Geometry check sheet. Reference: the model listing, model coordinates, mm. Face numbers are marked on the shaded views. A direction names the side the tool comes from. Coordinates: 2 decimals unless noted, no trailing zeros. Write each loop counter-clockwise with the first axis right and the second up, starting at its lowest first coordinate (ties: lowest second). Pieces come first, ordered by that corner, then holes.
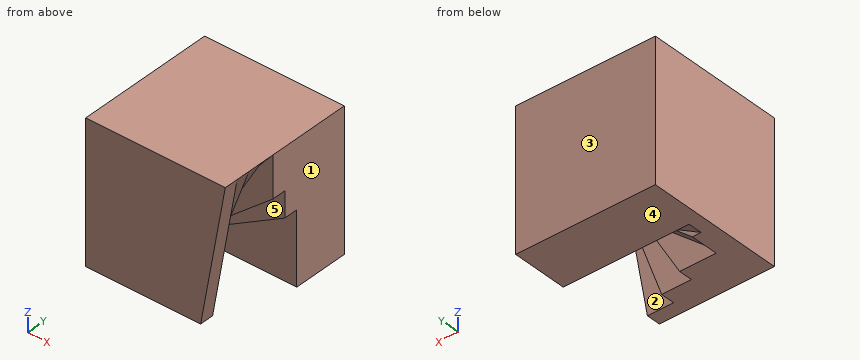
from build123d import *

# Parameters (mm, degrees)
F0_W      = 50.8
F0_H      = 50.8
F1_DEPTH  = 50.8
F3_DEPTH  = 5.08
F5_DEPTH  = 5.08
F7_DEPTH  = 5.08
F9_DEPTH  = 5.08
F11_DEPTH = 5.08
F13_DEPTH = 5.08


with BuildPart() as f1:
    # F0 (on Front) → F1 (new body)
    with BuildSketch(Plane.XZ):
        Rectangle(F0_W, F0_H)
    extrude(amount=F1_DEPTH)

    # F2 (on face) → F3 (cut)
    with BuildSketch(Plane.XZ.offset(50.8)):
        Polygon((31.007338, 25.4), (25.4, 25.4), (16.442589, -25.4), (31.007338, -25.4), align=None)
    extrude(amount=-F3_DEPTH, mode=Mode.SUBTRACT)

    # F4 (on face) → F5 (cut)
    with BuildSketch(Plane.XZ.offset(45.72)):
        Polygon((32.858667, 25.4), (25.4, 25.4), (6.626374, -26.180113), (32.858667, -26.180113), align=None)
    extrude(amount=-F5_DEPTH, mode=Mode.SUBTRACT)

    # F6 (on face) → F7 (cut)
    with BuildSketch(Plane.XZ.offset(40.64)):
        Polygon((35.186552, 25.4), (25.4, 25.4), (-7.151678, -30.981159), (35.186552, -30.981159), align=None)
    extrude(amount=-F7_DEPTH, mode=Mode.SUBTRACT)

    # F8 (on face) → F9 (cut)
    with BuildSketch(Plane.XZ.offset(35.56)):
        Polygon((63.193578, 25.4), (25.4, 25.4), (-24.735296, -34.348919), (63.193578, -34.348919), align=None)
    extrude(amount=-F9_DEPTH, mode=Mode.SUBTRACT)

    # F10 (on face) → F11 (cut)
    with BuildSketch(Plane.XZ.offset(30.48)):
        Polygon((66.855003, 25.4), (43.346025, 25.4), (-33.323239, -38.933151), (66.855003, -38.933151), align=None)
    extrude(amount=-F11_DEPTH, mode=Mode.SUBTRACT)

    # F12 (on face) → F13 (cut)
    with BuildSketch(Plane.XZ.offset(25.4)):
        Polygon((62.784301, 12.176968), (44.699044, 12.176968), (-34.901336, -33.780333), (62.784301, -33.780333), align=None)
    extrude(amount=-F13_DEPTH, mode=Mode.SUBTRACT)


solid = f1.part
1. Access from +Z, -Z, +X, -X, +Y, -Y to the whole of each face (thin tool, end or side, straight path). Record for the marked faces 1 and 2.
Computed values:
face 1: +Z, -Z, +X, +Y, -Y
face 2: -Z, +X
2. Draft check along Y on the marked faces 3, 4 and 5. Enter one of: released by +Y, released by -Y, zero draft, split by the parting line, or undercut.
Computed values:
face 3: released by +Y
face 4: zero draft
face 5: undercut
3. Sectioned sample at D-D, the plane x = 19. Record the boundary of the cut face in (y, z), and give its area (3 significant figures).
Computed values:
outline: (-50.8, -10.9) - (-45.72, -10.9) - (-45.72, 7.82) - (-40.64, 7.82) - (-40.64, 14.31) - (-35.56, 14.31) - (-35.56, 17.77) - (-30.48, 17.77) - (-30.48, 4.97) - (-25.4, 4.97) - (-25.4, -2.66) - (-20.32, -2.66) - (-20.32, -25.4) - (0, -25.4) - (0, 25.4) - (-50.8, 25.4) - close
area: 1,650 mm2
4. Gauge pin test, flat ends, axial feed: pin 1 Ø1.5 at (x, y) = (7, -28) entering from -Z; pin 2 Ø10 at (y, z) = (-42.5, 5.5) entering from +X. Record the tip position at first contact, or that the pin passes through.
Computed values:
pin 1: stops at z = -5.73
pin 2: stops at x = 22.57
5. Thickness scan on line 1 along Y through (x, z) = (19, -6.5); line 2 along Y through (x, z) = (-0.5, -10); line 3 along Y through (x, z) = (21, -8). Record the ranges inside material, lowest first.
Computed values:
line 1: y = -50.8 to -45.72, -20.32 to 0
line 2: y = -50.8 to -35.56, -30.48 to 0
line 3: y = -20.32 to 0
6. Sectioned sample at A-A, the plane x = -7.5. Record the boundary of the cut face in (y, z), and give its area (3 significant figures).
Computed values:
outline: (-50.8, -25.4) - (-35.56, -25.4) - (-35.56, -13.81) - (-30.48, -13.81) - (-30.48, -17.26) - (-25.4, -17.26) - (-25.4, -17.96) - (-20.32, -17.96) - (-20.32, -25.4) - (0, -25.4) - (0, 25.4) - (-50.8, 25.4) - close
area: 2,440 mm2
7. Sectioned sample at B-B, the plane z = 16.5. Record the boundary of the cut face in (x, y).
Computed values:
outline: (-25.4, -50.8) - (23.83, -50.8) - (23.83, -45.72) - (22.16, -45.72) - (22.16, -40.64) - (20.26, -40.64) - (20.26, -35.56) - (17.93, -35.56) - (17.93, -30.48) - (25.4, -30.48) - (25.4, 0) - (-25.4, 0) - close
8. Sectioned sample at C-C, the plane y = -48. Record the boundary of the cut face in (x, z).
Computed values:
outline: (-25.4, -25.4) - (16.44, -25.4) - (25.4, 25.4) - (-25.4, 25.4) - close
